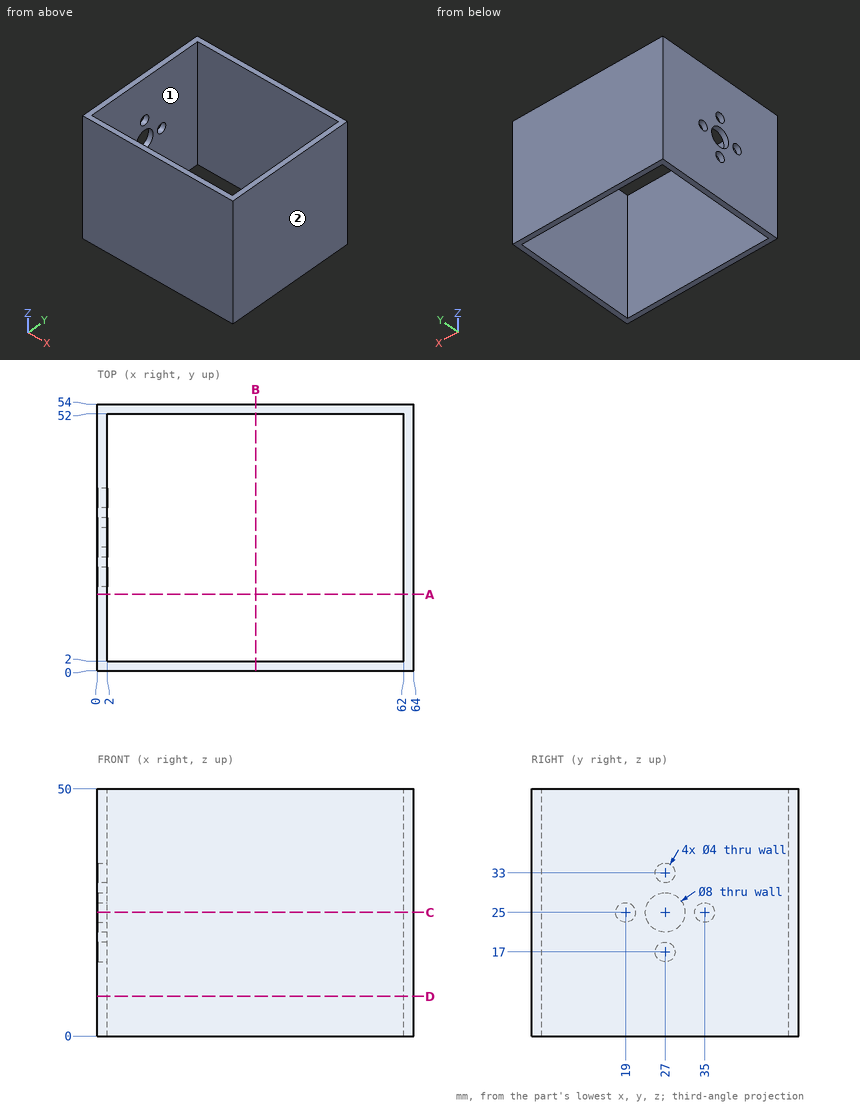
The drawing under review shows one solid part. Ordinate dimensions are in mm from its lowest x, y, z. A direction names the side the tool comes from. Coordinates: 2 decimals unless noted, no trailing zeros. Loops run counter-clockwise (first coordinate to the right, second up) from the corner with the lowest first, then second, coordinate; pieces in that order, holes last. Notation, with made-up numbers: (47.5, 31) - (105.5, 31) arc R21 ccw to (105.5, 35) - close; hole circle Ø1 at (-36.5, -27). An arc over 180 degrees is marked (long way). Use CSV: the item, a comma, the result in double quotes. Start each with the question number.
1. To check wall thickness, follow probe 1 along Y at (x, z) = (1, 25); probe 2 along Y at (x, z) = (49.5, 24); probe 3 along X at (y, z) = (16, 14). State the ranges of each line that lie inside material, in increasing order.
2. Clearance check with a flat-ended pin moving along its axis: pin 1 (3.5 mm diameter, centred on y = 27, z = 33, fed in from -X). State where the tip first meets the part, or that it passes through.
3. Add section C-C on z = 25. Give the boundary of the cut face in (x, y), plus the area to 3 significant figures.
4. Add section B-B on x = 32. Give the boundary of the cut face in (y, z).
5. Add section A-A on y = 15.5. Give the boundary of the cut face in (x, z).
6. For the marked faces 1 and 2, list the 3-axis set-ups (+Z, -Z, +X, -X, +Y, -Y) from which the entire face can be reached by the end or side of a thin tool; tool diameter is ignored.
7. Add section D-D on z = 8. Give the boundary of the cut face in (x, y), plus the area to 3 significant figures.
Resolved:
1,probe 1,"0 to 17, 21 to 23, 31 to 33, 37 to 54"
1,probe 2,"0 to 2, 52 to 54"
1,probe 3,"0 to 2, 62 to 64"
2,pin 1,"x = 62"
3,outline,"(0, 0) - (64, 0) - (64, 54) - (0, 54) - (0, 37) - (2, 37) - (2, 52) - (62, 52) - (62, 2) - (2, 2) - (2, 17) - (0, 17) - close; (0, 21) - (2, 21) - (2, 23) - (0, 23) - close; (0, 31) - (2, 31) - (2, 33) - (0, 33) - close"
3,area,"424 mm2"
4,outline,"(0, 0) - (2, 0) - (2, 50) - (0, 50) - close; (52, 0) - (54, 0) - (54, 50) - (52, 50) - close"
5,outline,"(0, 0) - (2, 0) - (2, 50) - (0, 50) - close; (62, 0) - (64, 0) - (64, 50) - (62, 50) - close"
6,face 1,"+Z, -Z"
6,face 2,"+Z, -Z, +X, +Y, -Y"
7,outline,"(0, 0) - (64, 0) - (64, 54) - (0, 54) - close; hole (2, 2) - (62, 2) - (62, 52) - (2, 52) - close"
7,area,"456 mm2"
